```python
from build123d import *

# Parameters (mm, degrees)
SKETCH1_R               = 18
BOSS_EXTRUDE1_DEPTH     = 20
SKETCH3_R               = 21
BOSS_EXTRUDE2_DEPTH     = 3
SKETCH4_R               = 21
BOSS_EXTRUDE3_DEPTH     = 3
CUT_EXTRUDE2_DEPTH      = 3
CUT_EXTRUDE2_DEPTH_BACK = 25
SKETCH6_R               = 1.5
CUT_EXTRUDE3_DEPTH      = 20


with BuildPart() as part:
    # Sketch1 → Boss-Extrude1 (new body)
    with BuildSketch(Plane(origin=(0, 0, 0), x_dir=(0, 0, -1), z_dir=(1, 0, 0))):
        Circle(SKETCH1_R)
    extrude(amount=BOSS_EXTRUDE1_DEPTH)

    # Sketch3 → Boss-Extrude2 (add)
    with BuildSketch(Plane(origin=(20, 0, 0), x_dir=(0, 0, -1), z_dir=(1, 0, 0))):
        Circle(SKETCH3_R)
    extrude(amount=BOSS_EXTRUDE2_DEPTH)

    # Sketch4 → Boss-Extrude3 (add)
    with BuildSketch(Plane.ZY):
        Circle(SKETCH4_R)
    extrude(amount=BOSS_EXTRUDE3_DEPTH)

    # Sketch2 → Cut-Extrude2 (cut, two sides)
    with BuildSketch(Plane(origin=(20, 0, 0), x_dir=(0, 0, -1), z_dir=(1, 0, 0))) as cut_extrude2_sk:
        with BuildLine():
            Line((-2.5, 13.609429768), (2.5, 13.609429768))
            Line((2.5, 13.609429768), (2.5, 10.766615067))
            ThreePointArc((2.5, 10.766615067), (2.542314031, 10.64359013), (2.651351351, 10.572622003))
            ThreePointArc((2.651351351, 10.572622003), (0, -10.9), (-2.651351351, 10.572622003))
            ThreePointArc((-2.651351351, 10.572622003), (-2.542314031, 10.64359013), (-2.5, 10.766615067))
            Line((-2.5, 10.766615067), (-2.5, 13.609429768))
        make_face()
    extrude(amount=CUT_EXTRUDE2_DEPTH, mode=Mode.SUBTRACT)
    extrude(cut_extrude2_sk.sketch, amount=-CUT_EXTRUDE2_DEPTH_BACK, mode=Mode.SUBTRACT)

    # Sketch6 → Cut-Extrude3 (cut)
    with BuildSketch(Plane.XZ.offset(-13.609429768)):
        with Locations((15, 0)):
            Circle(SKETCH6_R)
    extrude(amount=-CUT_EXTRUDE3_DEPTH, mode=Mode.SUBTRACT)


solid = part.part
```
CAD build for the part. Positions are in the model's coordinates, mm. A direction names the side the tool comes from. Coordinates: 2 decimals unless noted, no trailing zeros. Write each loop counter-clockwise with the first axis right and the second up, starting at its lowest first coordinate (ties: lowest second). Pieces come first, ordered by that corner, then holes. Notation, with made-up numbers: (-37, 7.25) -> (-25, 7.25) arc R17 ccw to (-25, 40.25) -> close; hole circle Ø4 at (17, 15.25). An arc over 180 degrees is marked (long way). Return JSON: item names as keys, results as strings. Group by question number.
Q1. Drill centre lines: line 1 (X direction, y = 15, z = 0); line 2 (Z direction, x = -2, y = 0.5); line 3 (Y direction, x = 2.5, z = 0). Where is each one in solid material? Low to high.
Q2. Cut at C-C, the plane x = 11.5. Give the cut face in (y, z).
Q3. Flat gauge pins, fed straight in: pin 1 (3 mm diameter, centred on x = 5.5, z = 15.5, fed in from +Y); pin 2 (2 mm diameter, centred on x = 5.5, z = 11.5, fed in from +Y); pin 3 (3.5 mm diameter, centred on x = 15, z = 0, fed in from -Y); pin 4 (13 mm diameter, centred on y = 0, z = 0, fed in from +X). Where does each tip first touch, or does it go through?
Q4. Pull direction Z, two halves, no side cores. Call faces 1 (the face through (-3, -9, 9)), 2 (the face through (-1.48, 6.31, 20.03)), 3 (the face through (10, 12, 2.5)), 4 (the face through (13.5, 15.77, 0.07)): released by +Z, released by -Z, zero draft, split by the parting line, or undercut.
Q5. Cut at D-D, the plane z = -6.5. Give the cut face in (x, y).
Q6. Cut at A-A, the plane y = 0. Give the cut face in (x, z), then the cut area to 3 significant figures.
Q7. Which spindle directions (+Z, -Z, +X, -X, +Y, -Y) get a long thin tool onto all of the face, cutting with end or side? Do faces 5 (the face through (23, -9, -9)), 6 (the face through (10, 13.609, 0)), 7 (the face through (0, 16, -9)). Say none if no direction does.
Q8. Cut at B-B, the plane z = 0. Give the cut face in (x, y), then the cut area to 3 significant figures.
Returned:
{
 "1": {"line 1": "x = -3 to 13.5, 16.5 to 23", "line 2": "z = -20.99 to -10.89, 10.89 to 20.99", "line 3": "y = -18 to -10.9, 13.61 to 18"},
 "2": {"outline": "circle Ø36 at (0, 0); hole (10.57, -2.65) arc R0.2 cw to (10.77, -2.5) -> (13.61, -2.5) -> (13.61, 2.5) -> (10.77, 2.5) arc R0.2 cw to (10.57, 2.65) arc R10.9 ccw (long way) to start"},
 "3": {"pin 1": "stops at y = 11.31", "pin 2": "stops at y = 14.62", "pin 3": "stops at y = -18", "pin 4": "passes through"},
 "4": {"face 1": "zero draft", "face 2": "split by the parting line", "face 3": "undercut", "face 4": "undercut"},
 "5": {"outline": "(-3, -19.97) -> (0, -19.97) -> (0, -16.79) -> (20, -16.79) -> (20, -19.97) -> (23, -19.97) -> (23, -8.75) -> (-3, -8.75) -> close; (-3, 8.75) -> (23, 8.75) -> (23, 19.97) -> (20, 19.97) -> (20, 16.79) -> (0, 16.79) -> (0, 19.97) -> (-3, 19.97) -> close"},
 "6": {"outline": "(-3, -21) -> (0, -21) -> (0, -18) -> (20, -18) -> (20, -21) -> (23, -21) -> (23, -10.9) -> (-3, -10.9) -> close; (-3, 10.9) -> (23, 10.9) -> (23, 21) -> (20, 21) -> (20, 18) -> (0, 18) -> (0, 21) -> (-3, 21) -> close", "area": "405 mm2"},
 "7": {"face 5": "+Z, -Z, +X, +Y, -Y", "face 6": "+X, -X", "face 7": "none"},
 "8": {"outline": "(-3, -21) -> (0, -21) -> (0, -18) -> (20, -18) -> (20, -21) -> (23, -21) -> (23, -10.9) -> (-3, -10.9) -> close; (-3, 13.61) -> (13.5, 13.61) -> (13.5, 18) -> (0, 18) -> (0, 21) -> (-3, 21) -> close; (16.5, 13.61) -> (23, 13.61) -> (23, 21) -> (20, 21) -> (20, 18) -> (16.5, 18) -> close", "area": "322 mm2"}
}
